Build history of the part. All positions in model axes, mm. Round coordinates to 2 decimals unless told otherwise and drop trailing zeros. Order: outer loops, then holes, each group sorted by start corner. A loop starts at its lowest first (then second) coordinate and runs counter-clockwise, first axis right, second up. Notation, with made-up numbers: (-22, 21) -> (-2, 21) arc R21 ccw to (-2, 39) -> close; hole circle Ø8 at (40, -12). An arc over 180 degrees is marked (long way). Use a Markdown table: item, result. Add a question column.
Item 1: Slice it at A-A, the plane x = 0. Give the cut face in (y, z), plus the area to 3 significant figures.
Item 2: Probe L1, parallel to Y at x = 0, z = 0.9; L2, parallel to X at y = -11, z = 1.15; L3, parallel to X at y = -13.5, z = 3.25. List the from-to ranges inside material, lowest first.
Item 3: Slice it at D-D, the plane y = -6.5. Give the cut face in (x, z).
Item 4: Slice it at B-B, the plane y = 0. Give the cut face in (x, z), plus the area to 3 significant figures.
Item 5: Pin check, flat tip, straight feed: pin 1 (4 mm diameter, centred on x = 12.12, y = 7, fed in from +Z). Stop position of the tip, or through.
Item 6: Two-plate mould, pull along X, no slides. Class faces 1 (the face through (8, -8, 0)), 2 (the face through (-13.887, -10.648, 1.972)), 3 (the face through (-10.785, 6.445, 1.014)): released by +X, released by -X, zero draft, split by the parting line, or undercut.
Item 7: Slice it at C-C, the plane z = 1.5. State how many separate pieces and enclosed holes the cut face has, plus the area to 3 significant figures.
from build123d import *

# Parameters (mm, degrees)
SKETCH1_R           = 17.5
BOSS_EXTRUDE1_DEPTH = 4
SKETCH2_R           = 10.5
CUT_EXTRUDE1_DEPTH  = 26.069902273
SKETCH3_R           = 1.6
CUT_EXTRUDE2_DEPTH  = 26.069902273
SKETCH4_R           = 1.45
CUT_EXTRUDE3_DEPTH  = 26.069902273
CHAMFER1_SIZE       = 2


with BuildPart() as part:
    # Sketch1 → Boss-Extrude1 (new body)
    with BuildSketch(Plane.XY):
        Circle(SKETCH1_R)
    extrude(amount=BOSS_EXTRUDE1_DEPTH)

    # Sketch2 → Cut-Extrude1 (cut, through all)
    with BuildSketch(Plane.XY.offset(4)):
        Circle(SKETCH2_R)
    extrude(amount=-CUT_EXTRUDE1_DEPTH, mode=Mode.SUBTRACT)

    # Sketch3 → Cut-Extrude2 (cut, through all)
    with BuildSketch(Plane.XY.offset(4)):
        with Locations((14, 0)):
            Circle(SKETCH3_R)
        with Locations((7, -12.124355653)):
            Circle(SKETCH3_R)
        with Locations((-7, -12.124355653)):
            Circle(SKETCH3_R)
        with Locations((-14, 0)):
            Circle(SKETCH3_R)
        with Locations((-7, 12.124355653)):
            Circle(SKETCH3_R)
        with Locations((7, 12.124355653)):
            Circle(SKETCH3_R)
    extrude(amount=-CUT_EXTRUDE2_DEPTH, mode=Mode.SUBTRACT)

    # Sketch4 → Cut-Extrude3 (cut, through all)
    with BuildSketch(Plane.XY.offset(4)):
        with Locations((12.124355653, 7)):
            Circle(SKETCH4_R)
        with Locations((0, -14)):
            Circle(SKETCH4_R)
        with Locations((-12.124355653, 7)):
            Circle(SKETCH4_R)
    extrude(amount=-CUT_EXTRUDE3_DEPTH, mode=Mode.SUBTRACT)

    # Chamfer1
    chamfer1_edges = [part.edges().sort_by_distance(p)[0] for p in [
        (10.674355653, 7, 4),
        (-1.45, -14, 4),
        (-13.574355653, 7, 4),
    ]]
    chamfer(chamfer1_edges, length=CHAMFER1_SIZE)


solid = part.part
Check sheet entries:
| question | item | result |
|---|---|---|
| 1 | outline | (-17.5, 0) -> (-15.45, 0) -> (-15.45, 2) -> (-17.45, 4) -> (-17.5, 4) -> close; (-12.55, 0) -> (-10.5, 0) -> (-10.5, 4) -> (-10.55, 4) -> (-12.55, 2) -> close; (10.5, 0) -> (17.5, 0) -> (17.5, 4) -> (10.5, 4) -> close |
| 1 | area | 40.4 mm2 |
| 2 | L1 | -17.5 to -15.45, -12.55 to -10.5, 10.5 to 17.5 |
| 2 | L2 | -13.61 to -8.14, -5.86 to 5.86, 8.14 to 13.61 |
| 2 | L3 | -11.14 to -7.82, -6.18 to -2.65, 2.65 to 6.18, 7.82 to 11.14 |
| 3 | outline | (-16.25, 0) -> (-8.25, 0) -> (-8.25, 4) -> (-16.25, 4) -> close; (8.25, 0) -> (16.25, 0) -> (16.25, 4) -> (8.25, 4) -> close |
| 4 | outline | (-17.5, 0) -> (-15.6, 0) -> (-15.6, 4) -> (-17.5, 4) -> close; (-12.4, 0) -> (-10.5, 0) -> (-10.5, 4) -> (-12.4, 4) -> close; (10.5, 0) -> (12.4, 0) -> (12.4, 4) -> (10.5, 4) -> close; (15.6, 0) -> (17.5, 0) -> (17.5, 4) -> (15.6, 4) -> close |
| 4 | area | 30.4 mm2 |
| 5 | pin 1 | z = 2.55 |
| 6 | face 1 | zero draft |
| 6 | face 2 | split by the parting line |
| 6 | face 3 | undercut |
| 7 | separate pieces | 1 |
| 7 | enclosed holes | 10 |
| 7 | area | 548 mm2 |
